Source: CAD feature listing. Evaluate the final solid. Frame: model axes, mm. Coordinates: 2 decimals unless noted, no trailing zeros. Order: outer loops, then holes, each group sorted by start corner. A loop starts at its lowest first (then second) coordinate and runs counter-clockwise, first axis right, second up.
Item 1: Ray query, line 1 (Z direction, x = -64.5, y = -5.5); line 2 (Y direction, x = -53, z = -5); line 3 (Z direction, x = 32.5, y = -7.5). Return the intervals inside material, ascending.
Item 2: Section C-C on z = -1.5. Return the cut outline in (x, y).
Item 3: Section A-A on x = -57.5. Return the cut outline in (y, z), then the cut area to 3 significant figures.
Item 4: Section B-B on y = -7. Return the cut outline in (x, z), then the cut area to 3 significant figures.
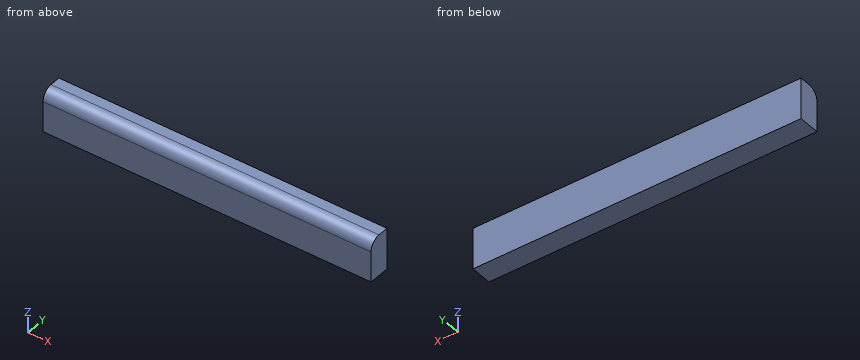
from build123d import *

# Parameters (mm, degrees)
F1_DEPTH = 10.16
F2_R     = 5.08


with BuildPart() as f1:
    # F0 (on Front) → F1 (new body)
    with BuildSketch(Plane.XZ):
        Polygon((77.562474, 0), (0, 0), (-78.607082, 0), (-78.607082, -19.587653), (77.562474, -19.587653), align=None)
    extrude(amount=F1_DEPTH)

    # F2
    f2_edges = [f1.edges().sort_by_distance(p)[0] for p in [
        (-0.522304, -10.16, 0),
    ]]
    fillet(f2_edges, radius=F2_R)


solid = f1.part
Answer list:
1. line 1: z = -19.59 to -0.02
1. line 2: y = -10.16 to 0
1. line 3: z = -19.59 to -0.61
2. outline: (-78.61, -8.68) - (77.56, -8.68) - (77.56, 0) - (-78.61, 0) - close
3. outline: (-10.16, -19.59) - (0, -19.59) - (0, 0) - (-5.08, 0) arc R5.08 ccw to (-10.16, -5.08) - close
3. area: 193 mm2
4. outline: (-78.61, -19.59) - (77.56, -19.59) - (77.56, -0.38) - (-78.61, -0.38) - close
4. area: 3,000 mm2
